from build123d import *

# Parameters (mm, degrees)
F0_W     = 25.4
F0_H     = 25.4
F1_DEPTH = 304.8
F3_D     = 5


with BuildPart() as f1:
    # F0 (on Front) → F1 (new body)
    with BuildSketch(Plane.XZ):
        Rectangle(F0_W, F0_H)
    extrude(amount=F1_DEPTH)

    # F3 (through all)
    with Locations(Plane.YZ.offset(12.7)):
        with Locations((-285.75, 0), (-241.3, 0), (-196.85, 0), (-152.4, 0), (-107.95, 0), (-63.5, 0), (-19.05, 0)):
            Hole(F3_D / 2)


solid = f1.part
Geometry: final body of the model. Coordinates: model frame, mm. Give positions to 0.01 mm unless a question says otherwise; leave off trailing zeros. Order: outer loops, then holes, each group sorted by start corner. A loop starts at its lowest first (then second) coordinate and runs counter-clockwise, first axis right, second up. Notation, with made-up numbers: (-15, 5) - (17, 5) arc R9 ccw to (17, 9) - close; hole circle Ø2 at (-34.5, 75.25). An arc over 180 degrees is marked (long way). Use CSV: the item, a comma, the result in double quotes.
1. Mould query, pull axis Y, two halves, no side actions, for faces 1 (the face through (-0.18, -18.51, -2.44)), 2 (the face through (0, -150, 12.7)), 3 (the face through (0, -304.8, 0)). Classes: +Y half, -Y half, draft (parallel to the pull), parting line (faces both ways), or undercut.
Answers below:
face 1,"undercut"
face 2,"draft"
face 3,"-Y half"
2. Section query A-A (y = -19.05). Output: boundary loops of the cut face in (x, z), plus the area to 3 significant figures.
Answers below:
outline,"(-12.7, -12.7) - (12.7, -12.7) - (12.7, -2.5) - (-12.7, -2.5) - close; (-12.7, 2.5) - (12.7, 2.5) - (12.7, 12.7) - (-12.7, 12.7) - close"
area,"518 mm2"
3. Contact query for a flat-ended pin moving along its axis: pin 1 (4 mm diameter, centred on y = -19.05, z = 0, fed in from -X). Output: stop coordinate, or through.
Answers below:
pin 1,"through"
4. Material intervals for line 1 along Z through (x, y) = (4.75, -19.05); line 2 along Z through (x, y) = (-5.75, -243.5), sorted ascending. Write a range as from..to.
Answers below:
line 1,"-12.7..-2.5, 2.5..12.7"
line 2,"-12.7..-1.19, 1.19..12.7"
5. Section query B-B (x = -2.5). Output: boundary loops of the cut face in (y, z).
Answers below:
outline,"(-304.8, -12.7) - (0, -12.7) - (0, 12.7) - (-304.8, 12.7) - close; hole circle Ø5 at (-285.75, 0); hole circle Ø5 at (-241.3, 0); hole circle Ø5 at (-196.85, 0); hole circle Ø5 at (-152.4, 0); hole circle Ø5 at (-107.95, 0); hole circle Ø5 at (-63.5, 0); hole circle Ø5 at (-19.05, 0)"
